from build123d import *

# Parameters (mm, degrees)
F1_DEPTH = 10
F4_SIZE  = 1


# Not quite as in the source:
# - a feature of the source that left no trace in its solid (it failed there, or was rolled back) is left out


with BuildPart() as f1:
    # F0 (on Front) → F1 (new body)
    with BuildSketch(Plane.XZ):
        Polygon((0, -25.5473433032), (0, -31.1332004264), (25.5, -31.1332004264), (21.4898194077, 10.9762813041), (42.9413538213, 4.1879331029), (42.9413538213, 36.1879331029), (31.0413538213, 36.1879331029), align=None)
    extrude(amount=F1_DEPTH)

    # F4
    f4_edges = [f1.edges().sort_by_distance(p)[0] for p in [
        (23.49491, 0, -10.07846),
        (32.215587, 0, 7.582107),
        (42.941354, 0, 20.187933),
        (15.520677, 0, 5.320295),
        (23.49491, -10, -10.07846),
        (32.215587, -10, 7.582107),
        (42.941354, -10, 20.187933),
        (15.520677, -10, 5.320295),
        (12.75, 0, -31.1332),
        (12.75, -10, -31.1332),
    ]]
    chamfer(f4_edges, length=F4_SIZE)


solid = f1.part
The model under review builds one solid part; all positions refer to its coordinate system, in mm. A direction names the side the tool comes from. Round coordinates to 2 decimals unless told otherwise and drop trailing zeros. Order: outer loops, then holes, each group sorted by start corner. A loop starts at its lowest first (then second) coordinate and runs counter-clockwise, first axis right, second up. Notation, with made-up numbers: (22, 31) -> (74, 31) arc R18 cw to (74, 40) -> close; hole circle Ø6 at (74.5, 74). An arc over 180 degrees is marked (long way). Write item = value, one per line. Start each with the question number.
Item 1: Clearance check with flat-ended pins moving along their axes: pin 1 Ø3 at (y, z) = (-1.5, -4) entering from -X; pin 2 Ø5 at (y, z) = (-2.5, -19) entering from -X; pin 3 Ø6 at (x, y) = (33, -7.5) entering from -Z. State where each tip first meets the part, or that it passes through.
Item 2: Consider section B-B on y = -7.5. Write out the cut boundary in (x, z).
Item 3: For line 1 along X through (y, z) = (-2, -28); line 2 along X through (y, z) = (-8.5, -25); line 3 along Z through (x, y) = (35.5, -7.25), list the stretches that pass through material, from the lowest coordinate up.
Item 4: Consider section D-D on z = -24.5. Write out the cut boundary in (x, y).
Item 5: Mouldability with a two-part tool opening along X and no side actions: class faces 1 (the face through (42.941, -5, 20)), 2 (the face through (31.488, -9.507, 8.344)), 3 (the face through (21, -10, 3)), 4 (the face through (0, -5, -28)) as released by +X, released by -X, zero draft, split by the parting line, or undercut.
Item 6: Consider section A-A on z = 9. Write out the cut boundary in (x, y), plus the area to 3 significant figures.
Item 7: Consider section C-C on x = 10.5. Write out the cut boundary in (y, z), plus the area to 3 significant figures.
Item 8: For faces 5 (the face through (32.07, -4.94, 7.63)), 6 (the face through (31.488, -0.493, 8.344)), 7 (the face through (22.948, -9.507, -9.68)), list the 3-axis set-ups (+Z, -Z, +X, -X, +Y, -Y) from which the entire face can be reached by the end or side of a thin tool; tool diameter is ignored.
Conclusion:
q1.pin_1 = 10.08
q1.pin_2 = 2.04
q1.pin_3 = 6.38
q2.outline = (0, -31.13) -> (25.5, -31.13) -> (21.49, 10.98) -> (42.94, 4.19) -> (42.94, 36.19) -> (31.04, 36.19) -> (0, -25.55) -> close
q3.line_1 = 0 to 25.2
q3.line_2 = 0.28 to 24.92
q3.line_3 = 6.54 to 36.19
q4.outline = (0.53, -9) -> (1.65, -10) -> (23.86, -10) -> (24.87, -9) -> (24.87, -1) -> (23.86, 0) -> (1.65, 0) -> (0.53, -1) -> close
q5.face_1 = released by +X
q5.face_2 = undercut
q5.face_3 = zero draft
q5.face_4 = released by -X
q6.outline = (17.37, -9) -> (18.49, -10) -> (20.67, -10) -> (21.68, -9) -> (21.68, -1) -> (20.67, 0) -> (18.49, 0) -> (17.37, -1) -> close; (27.73, -9) -> (31.05, -10) -> (41.94, -10) -> (42.94, -9) -> (42.94, -1) -> (41.94, 0) -> (31.05, 0) -> (27.73, -1) -> close
q6.area = 189 mm2
q7.outline = (-10, -30.13) -> (-9, -31.13) -> (-1, -31.13) -> (0, -30.13) -> (0, -6.89) -> (-1, -4.66) -> (-9, -4.66) -> (-10, -6.89) -> close
q7.area = 261 mm2
q8.face_5 = +Y, -Y
q8.face_6 = +Y
q8.face_7 = -Y
